Input: part model. Units: mm. Frame: model coordinates. A direction names the side the tool comes from. Round coordinates to 2 decimals unless told otherwise and drop trailing zeros. Loops run counter-clockwise (first coordinate to the right, second up) from the corner with the lowest first, then second, coordinate; pieces in that order, holes last. Notation, with made-up numbers: (19, 26.5) -> (45, 26.5) arc R27 ccw to (45, 44.5) -> close; hole circle Ø9 at (19, 85). An arc over 180 degrees is marked (long way). Answer as a JSON object with one key per item and string values. Group by question number.
Item 1: Draft query along X for faces 1 (the flat face through (0, 8, 17.786)), 2 (the cylindrical face through (0, 18.4, 18.1)), 3 (the flat face through (-3.05, 13, 20)). Return one class per face: released by +X, released by -X, zero draft, split by the parting line, or undercut.
Item 2: Set-up query: faces 4 (the cylindrical face through (-1.5, 14.5, 19.7)), 5 (the flat face through (-1, 16, 22)), 6 (the flat face through (3.05, 13, 20)). Return all of +Z, -Z, +X, -X, +Y, -Y with unobstructed straight access to the full face (end or side cutting, diameter ignored); none if empty.
Item 3: Section query D-D on z = 20.25. Return loops of the section in (x, y).
Item 4: Material intervals for line 1 (Z direction, x = 0, y = 11.5); line 2 (X direction, y = 16, z = 21.4); line 3 (X direction, y = 12.5, z = 20.1), sorted ascending. Write a range as [from, to].
Item 5: Section query C-C on z = 18. Return loops of the section in (x, y), and give its area (3 significant figures).
Item 6: Section query A-A on x = 0. Return loops of the section in (y, z), and give its area (3 significant figures).
Item 7: Pin query (flat end, axial travel): pin 1 (2.5 mm diameter, centred on x = 0, z = 19.77, fed in from +Y); pin 2 (2 mm diameter, centred on x = -0.5, y = 8, fed in from -Z). Return the tip coordinate at first contact, or that it passes through.
Item 8: Section query B-B on y = 16.5. Return loops of the section in (x, z).
Autodesk Inventor part; units mm, degrees
ref_plane "YZ Plane" through (0, 0, 0) normal (1, 0, 0) x (0, 1, 0)
ref_plane "XZ Plane" through (0, 0, 0) normal (0, 1, 0) x (-1, 0, 0)
ref_plane "XY Plane" through (0, 0, 0) normal (0, 0, 1) x (1, 0, 0)
sketch "Sketch1" plane through (0, 0, 0) normal (0, 1, 0) x (-1, 0, 0)
  line L0 (3.05, -5.3255) -> (-3.05, -5.3255)
  line L1 (-3.05, -5.3255) -> (-3.05, 4.8245)
  line L2 (-3.05, 4.8245) -> (3.05, 4.8245)
  line L3 (3.05, 4.8245) -> (3.05, -5.3255)
  line L4 (0.9, 4.8245) -> (-0.9, 4.8245)
  line L5 (0.9, 4.8245) -> (0.9, -5.3255)
  line L6 (-0.9, 4.8245) -> (-0.9, -5.3255)
  circle A0 centre (0, 3.486) radius 0.8
  circle A1 centre (-0.0087, -3.8255) radius 0.8
  line L7 (0, 4.8245) -> (0, -5.3255)
  line L8 (-3.05, 0) -> (3.05, 0)
  point P0 (0, 0)
  dimension "d13" = 6.1
  dimension "d44" = 1.8
  dimension "d45" = 2.15
  dimension "d46" = 1.6
  dimension "d47" = 1.6
extrude "Extrusion1" add sketch "Sketch1" along normal blind 10.15 contours L0 L5 L8 L3 | L0 L7 A1 L8 L5 | L8 L5 L2 L3 | L0 L6 L8 L7 A1 | L8 L7 A0 L2 L5 | L0 L1 L8 L6 | L8 L6 L2 L7 A0 | L8 L1 L2 L6
sketch "Sketch11" plane through (-3.05, 0, 4.8245) normal (0, 0, 1) x (1, 0, 0)
  point P0 (3.05, 0)
extrude "Extrusion6" add sketch "Sketch1" against normal blind 1 contours L0 L7 A1 L8 L5 | L0 L6 L8 L7 A1 | L8 L7 A0 L2 L5 | L8 L6 L2 L7 A0
sketch "Sketch12" plane through (0, 10.15, 0) normal (0, 1, 0) x (1, 0, 0)
  circle A0 centre (0.0087, 3.8255) radius 1.265
  circle A1 centre (0, -3.486) radius 1.265
  circle A2 centre (0, -3.486) radius 0.8
  circle A3 centre (0.0087, 3.8255) radius 0.8
  point P0 (0, 0)
  dimension "d52" = 2.53
  dimension "d53" = 2.53
extrude "Extrusion7" cut sketch "Sketch12" against normal blind 1 contours A0 | A1 | A2 | A3
sketch "Sketch13" plane through (-3.05, 10.15, 4.8245) normal (0, 0, 1) x (1, 0, 0)
  line L0 (0, 0) -> (0, -4.15)
  line L1 (0, -10.15) -> (0, 0)
  line L2 (0, -4.15) -> (6.1, -4.15)
  line L3 (6.1, -10.15) -> (6.1, 0)
  line L4 (6.1, 0) -> (6.1, -4.15)
  line L5 (0, 0) -> (6.1, 0)
  point P0 (3.05, -10.15)
  dimension "d56" = 4.15
extrude "Extrusion8" add sketch "Sketch13" along normal blind 17
sketch "Sketch17" plane through (-3.05, 10.15, 21.8245) normal (0, 0, 1) x (1, 0, 0)
  line L0 (6.1, 0) -> (0, 0)
  line L1 (6.1, 0) -> (14.3904, 5.5919)
  line L2 (6.1, 0) -> (16.1, 0) construction
  line L3 (14.3904, 5.5919) -> (10.1964, 11.8097)
  line L4 (10.1964, 11.8097) -> (13.5955, 14.1024)
  line L5 (13.5955, 14.1024) -> (17.7894, 7.8846)
  line L6 (17.7894, 7.8846) -> (19.7132, 5.0325)
  line L7 (6.1, -10.15) -> (6.1, -4.15)
  line L8 (19.7132, 5.0325) -> (6.1, -4.15)
  line L9 (6.1, 0) -> (6.1, -4.15)
  point P0 (3.05, -10.15)
  dimension "d72" = 10
  dimension "d73" = 34
  dimension "d74" = 7.5
  dimension "d75" = 4.1
extrude "Extrusion12" [suppressed]
sketch "Sketch14" plane through (0, 10.15, 0) normal (0, 1, 0) x (1, 0, 0)
  line L0 (3.05, 5.3255) -> (3.05, -21.8245)
  line L1 (3.05, -21.8245) -> (3.05, -17.7145)
  line L2 (3.05, -17.7145) -> (-3.05, -17.7145)
  line L3 (-3.05, 5.3255) -> (-3.05, -21.8245)
  line L4 (-3.05, -21.8245) -> (3.05, -21.8245)
  point P0 (0, 0)
  dimension "d59" = 4.11
extrude "Extrusion9" add sketch "Sketch14" along normal blind 9.25
sketch "Sketch16" plane through (0, 19.4, 0) normal (0, 1, 0) x (1, 0, 0)
  circle A0 centre (0, -19.7695) radius 1.5
  line L0 (-3.05, -21.8245) -> (3.05, -21.8245)
  line L1 (3.05, -21.8245) -> (3.05, -17.7145)
  point P0 (0, 0)
  point P1 (0, -21.8245)
  dimension "d67" = 3
  dimension "d68" = 2.055
  dimension "d69" = 3.05
extrude "Extrusion11" cut sketch "Sketch16" against normal blind 10
sketch "Sketch15" plane through (-3.05, 10.15, 21.8245) normal (0, 0, 1) x (1, 0, 0)
  line L0 (3.05, 7.25) -> (3.05, 4.45) construction
  line L1 (6.1, 0) -> (6.1, 9.25)
  line L2 (2.05, 7.25) -> (2.05, 4.45)
  line L3 (4.05, 4.45) -> (4.05, 7.25)
  arc A0 (4.05, 7.25) -> (2.05, 7.25) centre (3.05, 7.25) ccw
  arc A1 (2.05, 4.45) -> (4.05, 4.45) centre (3.05, 4.45) ccw
  line L4 (0, 9.25) -> (6.1, 9.25)
  line L5 (3.05, 9.25) -> (3.05, 8.25)
  point P0 (3.05, -10.15)
  point P1 (3.05, 5.85)
  dimension "d62" = 1.4
  dimension "d63" = 2
  dimension "d64" = 3.05
  dimension "d94" = 2.05
  dimension "d97" = 1
extrude "Extrusion10" cut sketch "Sketch15" against normal through all
sketch "Sketch20" plane through (10.5455, 24.2524, 21.8245) normal (-0.5591929, 0.8290376, 0) x (0.8290376, 0.5591929, 0)
  circle A0 centre (-2.05, 2.05) radius 1.5
  line L0 (-4.1, 0) -> (-4.1, 4.1)
  line L1 (0, 0) -> (-4.1, 0)
  point P0 (-22.3044, 21.8245)
  point P1 (-2.05, 0)
  dimension "d82" = 3
  dimension "d83" = 2.05
  dimension "d84" = 2.05
extrude "Extrusion14" [suppressed]
sketch "Sketch18" plane through (-3.05, 10.15, 21.8245) normal (0, 0, 1) x (1, 0, 0)
  line L0 (12.6984, 11.7664) -> (14.2641, 9.4451) construction
  line L1 (11.973, 11.2771) -> (13.5387, 8.9558)
  line L2 (14.9895, 9.9344) -> (13.4238, 12.2557)
  arc A0 (13.4238, 12.2557) -> (11.973, 11.2771) centre (12.6984, 11.7664) ccw
  arc A1 (13.5387, 8.9558) -> (14.9895, 9.9344) centre (14.2641, 9.4451) ccw
  line L3 (19.7132, 5.0325) -> (13.5955, 14.1024)
  line L4 (10.1964, 11.8097) -> (13.5955, 14.1024)
  point P0 (3.05, -10.15)
  point P1 (13.4813, 10.6057)
  point P2 (12.2091, 12.4918)
  dimension "d78" = 1.4
  dimension "d79" = 1.75
  dimension "d89" = 0.56
  dimension "d90" = 2.05
extrude "Extrusion13" cut sketch "Sketch18" against normal blind 4.1
sketch "Sketch21" plane through (13.8787, 15.6447, 19.7745) normal (-0.5591929, 0.8290376, 0) x (0.8290376, 0.5591929, 0)
  circle A0 centre (0, 0) radius 0.868
  point P0 (-20.2544, 19.7745)
extrude "Extrusion15" [suppressed]
mirror "Mirror3" about plane through (0, 0, 0) normal (1, 0, 0) of "Extrusion13"
fillet "Fillet1" radius 1 2 edges at (3.05, 10.15, 6.1945) (-3.05, 10.15, 6.1945)
fillet "Fillet2" [suppressed]
fillet "Fillet3" radius 1 2 edges at (3.05, 6, 13.3245) (-3.05, 6, 13.3245)
sketch "Sketch33" plane through (-3.05, 10.15, 21.8245) normal (0, 0, 1) x (1, 0, 0)
  line L0 (4.05, 7.25) -> (4.05, 4.45)
  arc A0 (2.05, 4.45) -> (4.05, 4.45) centre (3.05, 4.45) ccw
  line L1 (2.05, 4.45) -> (2.05, 7.25)
  arc A1 (4.05, 7.25) -> (2.05, 7.25) centre (3.05, 7.25) ccw
  arc A2 (0, -3.15) -> (1, -4.15) centre (1, -3.15) ccw
  line L2 (1, -4.15) -> (5.1, -4.15)
  arc A3 (5.1, -4.15) -> (6.1, -3.15) centre (5.1, -3.15) ccw
  line L3 (6.1, -3.15) -> (6.1, 9.25)
  line L4 (0, 9.25) -> (6.1, 9.25)
  line L5 (0, -3.15) -> (0, 9.25)
  point P0 (3.05, -10.15)
extrude "Extrusion17" add sketch "Sketch33" along normal blind 0.5
sketch "Sketch36" plane through (0, 10.15, 0) normal (0, 1, 0) x (1, 0, 0)
  line L0 (3.05, -17.7145) -> (3.05, 5.3255)
  line L1 (-3.5916, 5.3255) -> (3.05, 5.3255)
  line L2 (3.05, 5.3255) -> (3.05, -17.7864)
  line L3 (3.05, -17.7864) -> (-3.5916, -17.7864)
  line L4 (-3.5916, -17.7864) -> (-3.5916, 5.3255)
  point P0 (0, 0)
  point P1 (3.05, 5.3255)
extrude "Extrusion18" cut sketch "Sketch36" against normal through all
sketch "Sketch22" plane through (0, 9.4, 19.7695) normal (0, 1, 0) x (1, 0, 0)
  circle A0 centre (0, 0) radius 1.5
  point P0 (0, 19.7695)
extrude "Extrusion16" [suppressed]
equation "\"d13\" = base_width"
equation "\"d45\" = -0.5 * d44 + 0.5 * d13"
equation "\"d4\" = base_length"
equation "\"base_width\" = 6.1"
equation "\"base_length\" = 10.15"
equation "\"base_screw_diameter\" = 1.5"
equation "\"base_screw_spacing_edge\" = 8.5"
equation "\"multi_angle\" = 34deg"
properties part number "reinforced_holder"
Solved:
{
 "1": {"face 1": "zero draft", "face 2": "undercut", "face 3": "released by -X"},
 "2": {"face 4": "+Y", "face 5": "+Z, -Z", "face 6": "+Z, -Z, +X, +Y, -Y"},
 "3": {"outline": "(-3.05, 7) arc R1 ccw to (-2.05, 6) -> (2.05, 6) arc R1 ccw to (3.05, 7) -> (3.05, 19.4) -> (1.42, 19.4) -> (1.42, 9.4) -> (-1.42, 9.4) -> (-1.42, 19.4) -> (-3.05, 19.4) -> close"},
 "4": {"line 1": "[17.71, 18.27], [21.27, 22.32]", "line 2": "[-3.05, -1], [1, 3.05]", "line 3": "[-3.05, -1.46], [1.46, 3.05]"},
 "5": {"outline": "(-3.05, 7) arc R1 ccw to (-2.05, 6) -> (2.05, 6) arc R1 ccw to (3.05, 7) -> (3.05, 19.4) -> (-3.05, 19.4) -> close; hole (-1, 14.6) arc R1 ccw to (1, 14.6) -> (1, 17.4) arc R1 ccw to (-1, 17.4) -> close", "area": "72.6 mm²"},
 "6": {"outline": "(6, 17.79) -> (10.15, 17.79) -> (10.15, 17.71) -> (13.6, 17.71) -> (13.6, 18.27) -> (9.4, 18.27) -> (9.4, 21.27) -> (13.6, 21.27) -> (13.6, 22.32) -> (6, 22.32) -> close; (18.4, 17.71) -> (19.4, 17.71) -> (19.4, 18.27) -> (18.4, 18.27) -> close; (18.4, 21.27) -> (19.4, 21.27) -> (19.4, 22.32) -> (18.4, 22.32) -> close", "area": "23.7 mm²"},
 "7": {"pin 1": "y = 9.4", "pin 2": "z = 17.79"},
 "8": {"outline": "(-3.05, 17.71) -> (-1, 17.71) -> (-1, 18.65) arc R1.5 cw to (-1, 20.89) -> (-1, 22.32) -> (-3.05, 22.32) -> close; (1, 17.71) -> (3.05, 17.71) -> (3.05, 22.32) -> (1, 22.32) -> (1, 20.89) arc R1.5 cw to (1, 18.65) -> close"}
}
